Input: part model. Units: mm. Frame: model coordinates. Coordinates: 2 decimals unless noted, no trailing zeros. Answer as CSV lines item,"result". Start each with the question number.
Item 1: Draft query along Z for faces 1 (the cylindrical face through (-153.25, 0.79, -36.38)), 2 (the flat face through (-72, 3, 19)). Return one class per face: +Z half, -Z half, draft (parallel to the pull), parting line (faces both ways), or undercut.
Item 2: First-contact query: pin 1 (3 mm diameter, centred on x = 10.44, z = -36.16, fed in from +Y); pin 2 (2 mm diameter, centred on x = -15.5, z = 66.5, fed in from -Y); pin 3 (5.5 mm diameter, centred on x = -151.56, z = -36.16, fed in from +Y). Flat tips, straight axial feed; report the tip coordinate or a pass-through.
Item 3: Material intervals for line 1 along X through (y, z) = (2.75, -34); line 2 along X through (y, z) = (2.25, -24); line 3 along X through (y, z) = (2.55, 40.5), sorted ascending.
from build123d import *

# Parameters (mm, degrees)
SKETCH1_W                                      = 170
SKETCH1_H                                      = 120
BOSS_EXTRUDE1_DEPTH                            = 3
CSK_FOR_M3_FLAT_HEAD_MACHINE_SCREW1_AT_2_COUNT = 2
CSK_FOR_M3_FLAT_HEAD_MACHINE_SCREW1_AT_2_PITCH = 162
CSK_FOR_M3_FLAT_HEAD_MACHINE_SCREW1_AT_3_COUNT = 2
CSK_FOR_M3_FLAT_HEAD_MACHINE_SCREW1_AT_3_PITCH = 196.946693295
CSK_FOR_M3_FLAT_HEAD_MACHINE_SCREW1_AT_4_COUNT = 2
CSK_FOR_M3_FLAT_HEAD_MACHINE_SCREW1_AT_4_PITCH = 112
FILLET2_R                                      = 1


with BuildPart() as part:
    # Sketch1 → Boss-Extrude1 (new body)
    with BuildSketch(Plane(origin=(0, 0, 0), x_dir=(1, 0, 0), z_dir=(0, 1, 0))):
        with Locations((-70.564356436, -19.841584158)):
            Rectangle(SKETCH1_W, SKETCH1_H)
    extrude(amount=BOSS_EXTRUDE1_DEPTH)

    # Sketch4 → CSK for M3 Flat Head Machine Screw1 (revolve, cut)
    with BuildSketch(Plane(origin=(-151.564356436, 3, -36.158415842), x_dir=(0, 0, 1), z_dir=(1, 0, 0))):
        Polygon((0, 0), (0, 3), (1.7, 3), (1.7, 1.45), (3.15, 0), align=None)
    csk_for_m3_flat_head_machine_screw1 = revolve(axis=Axis((-151.564356436, 9.35, -36.158415842), (0, -1, 0)), mode=Mode.SUBTRACT)

    # CSK for M3 Flat Head Machine Screw1 at 2: CSK for M3 Flat Head Machine Screw1 ×2
    with Locations(*[(i * CSK_FOR_M3_FLAT_HEAD_MACHINE_SCREW1_AT_2_PITCH, 0, 0) for i in range(1, CSK_FOR_M3_FLAT_HEAD_MACHINE_SCREW1_AT_2_COUNT)]):
        add(csk_for_m3_flat_head_machine_screw1, mode=Mode.SUBTRACT)

    # CSK for M3 Flat Head Machine Screw1 at 3: CSK for M3 Flat Head Machine Screw1 ×2
    with Locations(*[Vector(0.8225576032241401, 0, 0.5686817997598994) * (i * CSK_FOR_M3_FLAT_HEAD_MACHINE_SCREW1_AT_3_PITCH) for i in range(1, CSK_FOR_M3_FLAT_HEAD_MACHINE_SCREW1_AT_3_COUNT)]):
        add(csk_for_m3_flat_head_machine_screw1, mode=Mode.SUBTRACT)

    # CSK for M3 Flat Head Machine Screw1 at 4: CSK for M3 Flat Head Machine Screw1 ×2
    with Locations(*[(0, 0, i * CSK_FOR_M3_FLAT_HEAD_MACHINE_SCREW1_AT_4_PITCH) for i in range(1, CSK_FOR_M3_FLAT_HEAD_MACHINE_SCREW1_AT_4_COUNT)]):
        add(csk_for_m3_flat_head_machine_screw1, mode=Mode.SUBTRACT)

    # Fillet2
    # the kernel refuses this fillet: 1 mm, written as the material it takes off along each edge
    with BuildSketch(Plane(origin=(13.435643564, 2, -39.158415842), x_dir=(1, 0, 0), z_dir=(0, 0, -1))) as fillet2_piece_1_section:
        Polygon((0, 0), (FILLET2_R, 0), (FILLET2_R, -FILLET2_R), (0, -FILLET2_R), align=None)
    fillet2_piece_1 = extrude(amount=FILLET2_R, mode=Mode.PRIVATE)
    fillet2_piece_1 = fillet2_piece_1 - Plane(origin=(13.435643564, 2, -39.158415842), x_dir=(-0.7071067811865475, -0.7071067811865475, 0), z_dir=(0, 0, -1)) * Sphere(FILLET2_R, mode=Mode.PRIVATE)
    add(fillet2_piece_1, mode=Mode.SUBTRACT)
    with BuildSketch(Plane(origin=(13.435643564, 2, 78.841584158), x_dir=(0, 1, 0), z_dir=(1, 0, 0))) as fillet2_piece_2_section:
        Polygon((0, 0), (FILLET2_R, 0), (FILLET2_R, FILLET2_R), (0, FILLET2_R), align=None)
    fillet2_piece_2 = extrude(amount=FILLET2_R, mode=Mode.PRIVATE)
    fillet2_piece_2 = fillet2_piece_2 - Plane(origin=(13.435643564, 2, 78.841584158), x_dir=(0, -0.7071067811865475, -0.7071067811865475), z_dir=(1, 0, 0)) * Sphere(FILLET2_R, mode=Mode.PRIVATE)
    add(fillet2_piece_2, mode=Mode.SUBTRACT)
    with BuildSketch(Plane(origin=(-154.564356436, 2, -39.158415842), x_dir=(-1, 0, 0), z_dir=(0, 0, -1))) as fillet2_piece_3_section:
        Polygon((0, 0), (FILLET2_R, 0), (FILLET2_R, FILLET2_R), (0, FILLET2_R), align=None)
    fillet2_piece_3 = extrude(amount=FILLET2_R, mode=Mode.PRIVATE)
    fillet2_piece_3 = fillet2_piece_3 - Plane(origin=(-154.564356436, 2, -39.158415842), x_dir=(0.7071067811865475, -0.7071067811865475, 0), z_dir=(0, 0, -1)) * Sphere(FILLET2_R, mode=Mode.PRIVATE)
    add(fillet2_piece_3, mode=Mode.SUBTRACT)
    with BuildSketch(Plane(origin=(-154.564356436, 2, 78.841584158), x_dir=(0, 1, 0), z_dir=(-1, 0, 0))) as fillet2_piece_4_section:
        Polygon((0, 0), (FILLET2_R, 0), (FILLET2_R, -FILLET2_R), (0, -FILLET2_R), align=None)
    fillet2_piece_4 = extrude(amount=FILLET2_R, mode=Mode.PRIVATE)
    fillet2_piece_4 = fillet2_piece_4 - Plane(origin=(-154.564356436, 2, 78.841584158), x_dir=(0, -0.7071067811865475, -0.7071067811865475), z_dir=(-1, 0, 0)) * Sphere(FILLET2_R, mode=Mode.PRIVATE)
    add(fillet2_piece_4, mode=Mode.SUBTRACT)
    with BuildSketch(Plane(origin=(14.435643564, 3, -39.158415842), x_dir=(0, -1, 0), z_dir=(0, 0, 1)), Plane(origin=(-155.564356436, 3, 78.841584158), x_dir=(0, -1, 0), z_dir=(0, 0, -1))) as fillet2_piece_5:
        with BuildLine():
            CenterArc((FILLET2_R, -FILLET2_R), FILLET2_R, 90, 90)
            Line((0, -FILLET2_R), (0, 0))
            Line((0, 0), (FILLET2_R, 0))
        make_face()
    extrude(amount=118, mode=Mode.SUBTRACT)
    with BuildSketch(Plane(origin=(-154.564356436, 3, -40.158415842), x_dir=(0, -1, 0), z_dir=(1, 0, 0))) as fillet2_piece_6:
        with BuildLine():
            CenterArc((FILLET2_R, -FILLET2_R), FILLET2_R, 90, 90)
            Line((0, -FILLET2_R), (0, 0))
            Line((0, 0), (FILLET2_R, 0))
        make_face()
    extrude(amount=168, mode=Mode.SUBTRACT)
    with BuildSketch(Plane(origin=(-155.564356436, -2.5, -40.158415842), x_dir=(1, 0, 0), z_dir=(0, 1, 0)), Plane(origin=(-155.564356436, -2.5, 79.841584158), x_dir=(0, 0, -1), z_dir=(0, 1, 0))) as fillet2_piece_7:
        with BuildLine():
            CenterArc((FILLET2_R, -FILLET2_R), FILLET2_R, 90, 90)
            Line((0, -FILLET2_R), (0, 0))
            Line((0, 0), (FILLET2_R, 0))
        make_face()
    extrude(amount=4.5, mode=Mode.SUBTRACT)
    with BuildSketch(Plane(origin=(14.435643564, -2.5, -40.158415842), x_dir=(-1, 0, 0), z_dir=(0, 1, 0)), Plane(origin=(14.435643564, -2.5, 79.841584158), x_dir=(0, 0, -1), z_dir=(0, 1, 0))) as fillet2_piece_8:
        with BuildLine():
            CenterArc((FILLET2_R, FILLET2_R), FILLET2_R, 180, 90)
            Line((0, FILLET2_R), (0, 0))
            Line((0, 0), (FILLET2_R, 0))
        make_face()
    extrude(amount=4.5, mode=Mode.SUBTRACT)
    with BuildSketch(Plane(origin=(13.435643564, 3, 79.841584158), x_dir=(0, 0, -1), z_dir=(-1, 0, 0))) as fillet2_piece_9:
        with BuildLine():
            CenterArc((FILLET2_R, FILLET2_R), FILLET2_R, 180, 90)
            Line((0, FILLET2_R), (0, 0))
            Line((0, 0), (FILLET2_R, 0))
        make_face()
    extrude(amount=168, mode=Mode.SUBTRACT)


solid = part.part
Determined:
1,face 1,"undercut"
1,face 2,"draft"
2,pin 1,"passes through"
2,pin 2,"stops at y = 0"
2,pin 3,"stops at y = 2.6"
3,line 1,"x = -155.23 to -153.5, -149.63 to 8.5, 12.37 to 14.1"
3,line 2,"x = -155.53 to 14.4"
3,line 3,"x = -155.4 to 14.27"
